Read the model definition and answer for the solid it produces. Units are mm, in the model's axes. Coordinates: 2 decimals unless noted, no trailing zeros. Loops run counter-clockwise (first coordinate to the right, second up) from the corner with the lowest first, then second, coordinate; pieces in that order, holes last. Notation, with made-up numbers: (22.5, 42.5) - (71.5, 42.5) arc R7 cw to (71.5, 51.5) - close; hole circle Ø5 at (29.25, -11). An arc over 180 degrees is marked (long way). Use one line per item in the form item = value.
from build123d import *

# Parameters (mm, degrees)
EXTRUDE_1_DEPTH            = 3
F_2_2_2_2_DIAMETER_HOLE1_D = 2.2
FILLET_1_R                 = 1


with BuildPart() as part:
    # 草图1 → 凸台-拉伸1 (new body)
    with BuildSketch(Plane(origin=(0, 0, 0), x_dir=(1, 0, 0), z_dir=(0, 1, 0))):
        with BuildLine():
            Line((-7.5, 5), (7.5, 5))
            ThreePointArc((7.5, 5), (9.267766953, 4.267766953), (10, 2.5))
            Line((10, 2.5), (10, -2.5))
            ThreePointArc((10, -2.5), (9.267766953, -4.267766953), (7.5, -5))
            Line((7.5, -5), (-7.5, -5))
            ThreePointArc((-7.5, -5), (-9.267766953, -4.267766953), (-10, -2.5))
            Line((-10, -2.5), (-10, 2.5))
            ThreePointArc((-10, 2.5), (-9.267766953, 4.267766953), (-7.5, 5))
        make_face()
    extrude(amount=EXTRUDE_1_DEPTH)

    # Ø2.2 (2.2) Diameter Hole1 (through all)
    with Locations(Plane(origin=(0, 3, 0), x_dir=(1, 0, 0), z_dir=(0, 1, 0))):
        with Locations((-7.5, 0), (-2.5, 0)):
            f_2_2_2_2_diameter_hole1 = Hole(F_2_2_2_2_DIAMETER_HOLE1_D / 2)

    # 镜向1: Ø2.2 (2.2) Diameter Hole1 across plane
    add(f_2_2_2_2_diameter_hole1.mirror(Plane(origin=(0, 0, 0), x_dir=(0, 0, 1), z_dir=(1, 0, 0))), mode=Mode.SUBTRACT)

    # 圆角1
    fillet_1_edges = [part.edges().sort_by_distance(p)[0] for p in [
        (0, 0, -5),
        (9.267766953, 0, -4.267766953),
        (10, 0, 0),
        (9.267766953, 0, 4.267766953),
        (9.267766953, 3, -4.267766953),
        (0, 3, -5),
        (-9.267766953, 3, -4.267766953),
        (-10, 3, 0),
        (-9.267766953, 3, 4.267766953),
        (0, 3, 5),
        (9.267766953, 3, 4.267766953),
        (0, 0, 5),
        (10, 3, 0),
        (-9.267766953, 0, 4.267766953),
        (-10, 0, 0),
        (-9.267766953, 0, -4.267766953),
    ]]
    fillet(fillet_1_edges, radius=FILLET_1_R)


solid = part.part
Item 1: The part is cut by section D-D on x = -4. Give the vertices of the cut face in (y, z).
Results below:
outline = (0, -4) arc R1 ccw to (1, -5) - (2, -5) arc R1 ccw to (3, -4) - (3, 4) arc R1 ccw to (2, 5) - (1, 5) arc R1 ccw to (0, 4) - close
Item 2: Find the intervals of material crossed by L1, parallel to Z at x = -7.5, y = 2; L2, parallel to Z at x = 1.5, y = 1.15; L3, parallel to Y at x = 8.75, z = 3.75, in increasing order.
Results below:
L1 = -5 to -1.1, 1.1 to 5
L2 = -5 to -0.46, 0.46 to 5
L3 = 0.04 to 2.96
Item 3: The part is cut by section C-C on y = 1.55. Give the vertices of the cut face in (x, z).
Results below:
outline = (-10, -2.5) arc R2.5 ccw to (-7.5, -5) - (7.5, -5) arc R2.5 ccw to (10, -2.5) - (10, 2.5) arc R2.5 ccw to (7.5, 5) - (-7.5, 5) arc R2.5 ccw to (-10, 2.5) - close; hole circle Ø2.2 at (-7.5, 0); hole circle Ø2.2 at (-2.5, 0); hole circle Ø2.2 at (2.5, 0); hole circle Ø2.2 at (7.5, 0)
Item 4: The part is cut by section A-A on z = 0. Give the vertices of the cut face in (x, y).
Results below:
outline = (-10, 1) arc R1 ccw to (-9, 0) - (-8.6, 0) - (-8.6, 3) - (-9, 3) arc R1 ccw to (-10, 2) - close; (-6.4, 0) - (-3.6, 0) - (-3.6, 3) - (-6.4, 3) - close; (-1.4, 0) - (1.4, 0) - (1.4, 3) - (-1.4, 3) - close; (3.6, 0) - (6.4, 0) - (6.4, 3) - (3.6, 3) - close; (8.6, 0) - (9, 0) arc R1 ccw to (10, 1) - (10, 2) arc R1 ccw to (9, 3) - (8.6, 3) - close
Item 5: The part is cut by section B-B on x = 2.5. Give the vertices of the cut face in (y, z).
Results below:
outline = (0, -4) arc R1 ccw to (1, -5) - (2, -5) arc R1 ccw to (3, -4) - (3, -1.1) - (0, -1.1) - close; (0, 1.1) - (3, 1.1) - (3, 4) arc R1 ccw to (2, 5) - (1, 5) arc R1 ccw to (0, 4) - close
Item 6: This flat-tipped pin is pushed along its axis until it touches: P1, Ø3, axis at x = 7.5, z = 0, coming from the +Y side. Where does it stop, or does it pass through?
Results below:
P1 = 3
Item 7: For a pull along X with two mould halves and no side action, classify faces 1 (the cylindrical face through (9.715, 0.301, 0.035)), 2 (the cylindrical face through (-3.55, 1.48, -0.33)), 3 (the cylindrical face through (0.105, 0.301, -4.715)) as +X half, -X half, draft (parallel to the pull), parting line (faces both ways), or undercut.
Results below:
face_1 = +X half
face_2 = undercut
face_3 = draft
